Input: part model. Units: mm. Frame: model coordinates. Face numbers are marked on the shaded views. Give positions to 0.01 mm unless a question says otherwise; leave off trailing zeros. Write each loop counter-clockwise with the first axis right and the second up, starting at its lowest first coordinate (ties: lowest second). Pieces come first, ordered by that corner, then holes. Notation, with made-up numbers: (25.5, 74.25) - (38.5, 74.25) arc R5 ccw to (38.5, 79.25) - close; hole circle Ø2 at (-32.75, 85). An arc over 180 degrees is marked (long way). Answer as a JSON object with one key per item and string values. Group by question number.
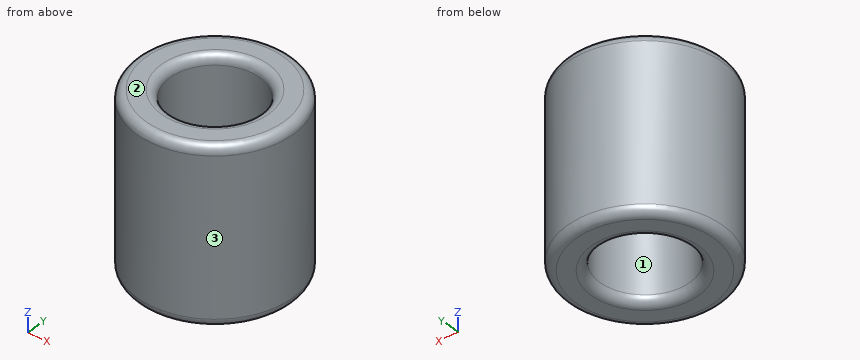
Solid Edge part; units mm, degrees
sketch "Sketch1" plane through (0, 0, 0) normal (0, 0, 1) x (1, 0, 0)
  circle A0 centre (0, 0) radius 4.5
  circle A1 centre (0, 0) radius 2.6
extrude "Protrusion1" add sketch "Sketch1" along normal mid plane 10
fillet "Round_1" radius 0.5 2 edges at (-2.6, 0, -5) (-2.6, 0, 5)
fillet "Round_2" radius 0.5 2 edges at (-4.5, 0, -5) (-4.5, 0, 5)
properties material "Acrylic, high impact grade"
1) Cut plane C-C on z = -4. Return the cut outline in (x, y).
2) Pin query (flat end, axial travel): P1, Ø1, axis at x = -2.5, z = -2.5, coming from the +Y side; P2, Ø1, axis at y = -1, z = -3, coming from the +X side; P3, Ø2, axis at y = 2.5, z = 2, coming from the +X side. Return the tip coordinate at first contact, or that it passes through.
3) Mould query, pull axis X, two halves, no side actions, for the marked faces 1, 2 and 3. Classes: +X half, -X half, draft (parallel to the pull), parting line (faces both ways), or undercut.
4) Cut plane A-A on x = 0. Return the cut outline in (y, z), and give its area (3 significant figures).
5) Line query: line 1 along Y through (x, z) = (0, 0.75); line 2 along X through (y, z) = (-2, -0.75); line 3 along Y through (x, z) = (-1.5, 2). Output: solid intervals per line, ascending. Write a range as from..to.
Filled in:
{
 "1": {"outline": "circle Ø9 at (0, 0); hole circle Ø5.2 at (0, 0)"},
 "2": {"P1": "stops at y = 4.03", "P2": "stops at x = 4.47", "P3": "stops at x = 4.24"},
 "3": {"face 1": "undercut", "face 2": "draft", "face 3": "parting line"},
 "4": {"outline": "(-4.5, -4.5) arc R0.5 ccw to (-4, -5) - (-3.1, -5) arc R0.5 ccw to (-2.6, -4.5) - (-2.6, 4.5) arc R0.5 ccw to (-3.1, 5) - (-4, 5) arc R0.5 ccw to (-4.5, 4.5) - close; (2.6, -4.5) arc R0.5 ccw to (3.1, -5) - (4, -5) arc R0.5 ccw to (4.5, -4.5) - (4.5, 4.5) arc R0.5 ccw to (4, 5) - (3.1, 5) arc R0.5 ccw to (2.6, 4.5) - close", "area": "37.6 mm²"},
 "5": {"line 1": "y = -4.5..-2.6, 2.6..4.5", "line 2": "x = -4.03..-1.66, 1.66..4.03", "line 3": "y = -4.24..-2.12, 2.12..4.24"}
}
